Input: part model. Units: mm. Frame: model coordinates. A direction names the side the tool comes from. Give positions to 0.01 mm unless a question says otherwise; leave off trailing zeros. Loops run counter-clockwise (first coordinate to the right, second up) from the corner with the lowest first, then second, coordinate; pieces in that order, holes last.
from build123d import *

# Parameters (mm, degrees)
SKETCH1_W                                            = 82.55
SKETCH1_H                                            = 41.4147
BOSS_EXTRUDE1_DEPTH                                  = 12.7
SKETCH2_R                                            = 3.175
CUT_EXTRUDE1_DEPTH                                   = 12.7
SKETCH3_R                                            = 8.89
CUT_EXTRUDE2_DEPTH                                   = 6.35
SKETCH5_R                                            = 10.414
CUT_EXTRUDE7_DEPTH                                   = 1.5875
FILLET1_R                                            = 2.54
CBORE_FOR_3_8_BINDING_HEAD_MACHINE_SCREW_D           = 10.0838
CBORE_FOR_3_8_BINDING_HEAD_MACHINE_SCREW_CBORE_D     = 20.6375
CBORE_FOR_3_8_BINDING_HEAD_MACHINE_SCREW_CBORE_DEPTH = 6.4262


with BuildPart() as part:
    # Sketch1 → Boss-Extrude1 (new body)
    with BuildSketch(Plane.XY):
        Rectangle(SKETCH1_W, SKETCH1_H)
    extrude(amount=BOSS_EXTRUDE1_DEPTH)

    # Sketch2 → Cut-Extrude1 (cut)
    with BuildSketch(Plane.XY.offset(12.7)):
        Circle(SKETCH2_R)
    extrude(amount=-CUT_EXTRUDE1_DEPTH, mode=Mode.SUBTRACT)

    # Sketch3 → Cut-Extrude2 (cut)
    with BuildSketch(Plane.XY.offset(12.7)):
        Circle(SKETCH3_R)
    extrude(amount=-CUT_EXTRUDE2_DEPTH, mode=Mode.SUBTRACT)

    # Sketch5 → Cut-Extrude7 (cut)
    with BuildSketch(Plane.XY.offset(12.7)):
        Circle(SKETCH5_R)
    extrude(amount=-CUT_EXTRUDE7_DEPTH, mode=Mode.SUBTRACT)

    # Fillet1
    fillet1_edges = [part.edges().sort_by_distance(p)[0] for p in [
        (41.275, -20.70735, 6.35),
        (-41.275, -20.70735, 6.35),
        (-41.275, 20.70735, 6.35),
        (41.275, 20.70735, 6.35),
    ]]
    fillet(fillet1_edges, radius=FILLET1_R)

    # CBORE for 3/8 Binding Head Machine Screw1 (through all)
    with Locations(Plane.XY.offset(12.7)):
        with Locations((-29, -6.708000046), (29, -6.708000046)):
            CounterBoreHole(CBORE_FOR_3_8_BINDING_HEAD_MACHINE_SCREW_D / 2, CBORE_FOR_3_8_BINDING_HEAD_MACHINE_SCREW_CBORE_D / 2, CBORE_FOR_3_8_BINDING_HEAD_MACHINE_SCREW_CBORE_DEPTH)


solid = part.part
(1) Pin query (flat end, axial travel): pin 1 Ø13 at (x, y) = (-29, -6.708) entering from +Z. Return the tip coordinate at first contact, or that it passes through.
Values follow:
pin 1: stops at z = 6.27
(2) Ray query, probe 1 along Y at (x, z) = (29, 8.25); probe 2 along X at (y, z) = (-7, 9.5) (3 decimals); probe 3 along X at (y, z) = (-6.5, 10.5) (3 decimals). Return the intervals inside material, ascending.
Values follow:
probe 1: y = -20.71 to -17.03, 3.61 to 20.71
probe 2: x = -41.275 to -39.315, -18.685 to -5.48, 5.48 to 18.685, 39.315 to 41.275
probe 3: x = -41.275 to -39.317, -18.683 to -6.065, 6.065 to 18.683, 39.317 to 41.275
(3) Reachability of faces 1 (the cylindrical face through (-1.93, -8.68, 8.76)), 2 (the cylindrical face through (40.511, -19.983, 6.439)) from +Z, -Z, +X, -X, +Y, -Y: full face, straight path, thin tool, end or side. Return the list, or none.
Values follow:
face 1: +Z
face 2: +Z, -Z, +X, -Y
(4) Cut plane A-A (x = -29). Return the cut outline in (y, z).
Values follow:
outline: (-20.71, 0) - (-11.75, 0) - (-11.75, 6.27) - (-17.03, 6.27) - (-17.03, 12.7) - (-20.71, 12.7) - close; (-1.67, 0) - (20.71, 0) - (20.71, 12.7) - (3.61, 12.7) - (3.61, 6.27) - (-1.67, 6.27) - close
(5) Cut plane D-D (y = -5). Count the separate pieces of the cut face and the enclosed holes in it, and give its area (3 significant figures).
Values follow:
separate pieces: 3
enclosed holes: 0
area: 569 mm2
(6) Mould query, pull axis Y, two halves, no side actions, for faces 3 (the flat face through (41.275, 0, 6)), 4 (the cylindrical face through (34.037, -6.486, 3.093)), 5 (the cylindrical face through (-40.551, 19.944, 6.439)). Classes: +Y half, -Y half, draft (parallel to the pull), parting line (faces both ways), or undercut.
Values follow:
face 3: draft
face 4: undercut
face 5: +Y half
